Read the model definition and answer for the solid it produces. Units are mm, in the model's axes. Coordinates: 2 decimals unless noted, no trailing zeros. Write each loop counter-clockwise with the first axis right and the second up, starting at its lowest first coordinate (ties: lowest second). Pieces come first, ordered by that corner, then holes. Notation, with made-up numbers: (1, 81) - (34, 81) arc R27 cw to (34, 112) - close; hole circle Ø10 at (-7, 84). An arc over 180 degrees is marked (long way). Use a Markdown table: item, result.
from build123d import *

# Parameters (mm, degrees)
ESBO_O1_R                = 5
RESSALTO_EXTRUS_O1_DEPTH = 63
SKETCH1_W                = 5
SKETCH1_H                = 14
CUT_EXTRUDE1_DEPTH       = 7


with BuildPart() as part:
    # Esboço1 → Ressalto-extrusão1 (new, symmetric)
    with BuildSketch(Plane.XY):
        with Locations((0, 100)):
            Circle(ESBO_O1_R)
    extrude(amount=RESSALTO_EXTRUS_O1_DEPTH, both=True)

    # Sketch1 → Cut-Extrude1 (cut)
    with BuildSketch(Plane.XY.offset(63)):
        with Locations((3, 100)):
            Rectangle(SKETCH1_W, SKETCH1_H)
        with Locations((-3, 100)):
            Rectangle(SKETCH1_W, SKETCH1_H)
    extrude(amount=-CUT_EXTRUDE1_DEPTH, mode=Mode.SUBTRACT)


solid = part.part
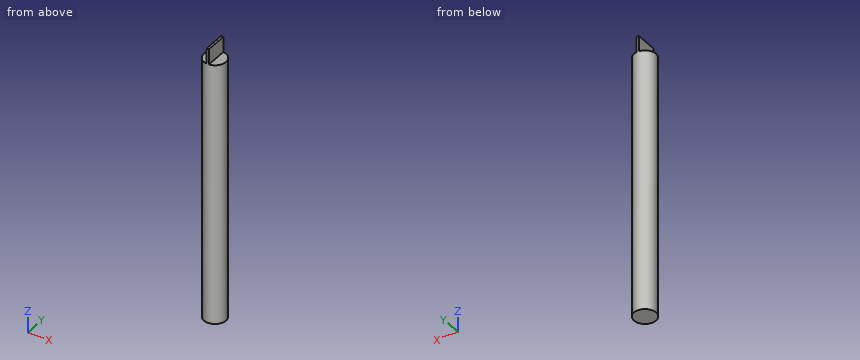
(1) A cutting plane is placed at B-B, the plane z = 49. Write down the section's boundary in (x, y), and give its area (3 significant figures).
Report:
| item | result |
|---|---|
| outline | circle Ø10 at (0, 100) |
| area | 78.5 mm² |
(2) Straight lines are drawn through the part: L1, parallel to X at y = 100.5, z = -26; L2, parallel to Z at x = 4.25, y = 102.5; L3, parallel to Y at x = -0.5, z = 32.5. For each, find the intervals that lie inside material, in ascending order.
Report:
| item | result |
|---|---|
| L1 | x = -4.97 to 4.97 |
| L2 | z = -63 to 56 |
| L3 | y = 95.03 to 104.97 |
(3) A cutting plane is placed at A-A, the plane y = 100. Write down the section's boundary in (x, z).
Report:
| item | result |
|---|---|
| outline | (-5, -63) - (5, -63) - (5, 56) - (0.5, 56) - (0.5, 63) - (-0.5, 63) - (-0.5, 56) - (-5, 56) - close |
(4) A cutting plane is placed at C-C, the plane x = 2.5. Write down the section's boundary in (y, z).
Report:
| item | result |
|---|---|
| outline | (95.67, -63) - (104.33, -63) - (104.33, 56) - (95.67, 56) - close |
(5) Each of these flat-tipped pins is pushed along its axis until it touches: P1, Ø4, axis at y = 102.5, z = 27, coming from the +X side; P2, Ø2, axis at y = 102, z = 58, coming from the +X side; P3, Ø3.5, axis at x = -3.5, y = 99.5, coming from the +Z side. Where does it stop, or does it pass through?
Report:
| item | result |
|---|---|
| P1 | stops at x = 4.97 |
| P2 | stops at x = 0.5 |
| P3 | stops at z = 56 |
